Design review of the part built by this model. Coordinates are the model's own, in mm. A direction names the side the tool comes from. Coordinates: 2 decimals unless noted, no trailing zeros. Order: outer loops, then holes, each group sorted by start corner. A loop starts at its lowest first (then second) coordinate and runs counter-clockwise, first axis right, second up. Notation, with made-up numbers: (69.5, -26.75) -> (119.5, -26.75) arc R16 cw to (119.5, -1.75) -> close; hole circle Ø10 at (85.5, -10.75). An arc over 180 degrees is marked (long way). Write item = value, one per line.
```python
from build123d import *

# Parameters (mm, degrees)
IZIM1_R                     = 4.960788644
Y_KSEKLIK_EKSTR_ZYON1_DEPTH = 5


with BuildPart() as part:
    # Çizim1 → Yükseklik-Ekstrüzyon1 (new body)
    with BuildSketch(Plane(origin=(0, 0, 0), x_dir=(1, 0, 0), z_dir=(0, 1, 0))):
        with BuildLine():
            ThreePointArc((0, -15.612956291), (-15.612956291, 0), (0, 15.612956291))
            Line((0, 15.612956291), (36.486144355, 15.612956291))
            ThreePointArc((36.486144355, 15.612956291), (-39.686309151, 0), (36.486144355, -15.612956291))
            Line((36.486144355, -15.612956291), (0, -15.612956291))
        make_face()
        with Locations(Location((-28, -0.544306251, 0), (0, 0, 270))):
            Circle(IZIM1_R, mode=Mode.SUBTRACT)
        with Locations(Location((0, -28, 0), (0, 0, 270))):
            Circle(IZIM1_R, mode=Mode.SUBTRACT)
        with Locations(Location((0, 28, 0), (0, 0, 270))):
            Circle(IZIM1_R, mode=Mode.SUBTRACT)
    extrude(amount=Y_KSEKLIK_EKSTR_ZYON1_DEPTH)


solid = part.part
```
(1) We need section A-A (y = 3.5). Write out the cut boundary in (x, z).
Report:
outline = (0, -15.61) arc R15.61 cw to (0, 15.61) -> (36.49, 15.61) arc R39.69 ccw (long way) to (36.49, -15.61) -> close; hole circle Ø9.92 at (-28, 0.54); hole circle Ø9.92 at (0, -28); hole circle Ø9.92 at (0, 28)
(2) For faces 1 (the flat face through (18, 2, -15.613)), 2 (the cylindrical face through (1.49, 2.46, -23.27)), list the 3-axis set-ups (+Z, -Z, +X, -X, +Y, -Y) from which the entire face can be reached by the end or side of a thin tool; tool diameter is ignored.
Report:
face_1 = +X, +Y, -Y
face_2 = +Y, -Y
(3) We need section D-D (x = 3). Write out the cut boundary in (y, z), and give its area (3 significant figures).
Report:
outline = (0, -39.57) -> (5, -39.57) -> (5, -31.95) -> (0, -31.95) -> close; (0, -24.05) -> (5, -24.05) -> (5, -15.61) -> (0, -15.61) -> close; (0, 15.61) -> (5, 15.61) -> (5, 24.05) -> (0, 24.05) -> close; (0, 31.95) -> (5, 31.95) -> (5, 39.57) -> (0, 39.57) -> close
area = 161 mm²
(4) We need section C-C (x = -28). Write out the cut boundary in (y, z).
Report:
outline = (0, -28.12) -> (5, -28.12) -> (5, -4.42) -> (0, -4.42) -> close; (0, 5.51) -> (5, 5.51) -> (5, 28.12) -> (0, 28.12) -> close
(5) We need section B-B (z = -0.5). Write out the cut boundary in (x, y).
Report:
outline = (-39.68, 0) -> (-32.85, 0) -> (-32.85, 5) -> (-39.68, 5) -> close; (-23.15, 0) -> (-15.6, 0) -> (-15.6, 5) -> (-23.15, 5) -> close
(6) For L1, parallel to Z at x = -3.5, y = 1.05; L2, parallel to Z at x = 24.5, y = 3.65; L3, parallel to Z at x = -8.5, y = 0.9, list the stretches that pass through material, from the lowest coordinate up.
Report:
L1 = -39.53 to -31.52, -24.48 to -15.22, 15.22 to 24.48, 31.52 to 39.53
L2 = -31.22 to -15.61, 15.61 to 31.22
L3 = -38.77 to -13.1, 13.1 to 38.77
(7) The part is to be moulded in two halves that separate along X. For faces 3 (the cylindrical face through (-15.61, 2.46, 0.34)), 4 (the flat face through (18, 2, 15.613)), 5 (the cylindrical face through (-1.9, 2.465, 32.583)), say which applies: released by +X, released by -X, zero draft, split by the parting line, or undercut.
Report:
face_3 = released by +X
face_4 = zero draft
face_5 = undercut
(8) Insertion check: pin 1 (1 mm diameter, centred on y = 3.5, z = -29, fed in from -X); pin 2 (3 mm diameter, centred on x = 25, y = 1.5, fed in from +Z); pin 3 (1.5 mm diameter, centred on x = 15.5, y = 1.5, fed in from +Z). Each pin has a flat end and moves straight along its axis. Give the tip position at first contact, or say it passes through.
Report:
pin_1 = -27.62
pin_2 = 31.98
pin_3 = 36.84
